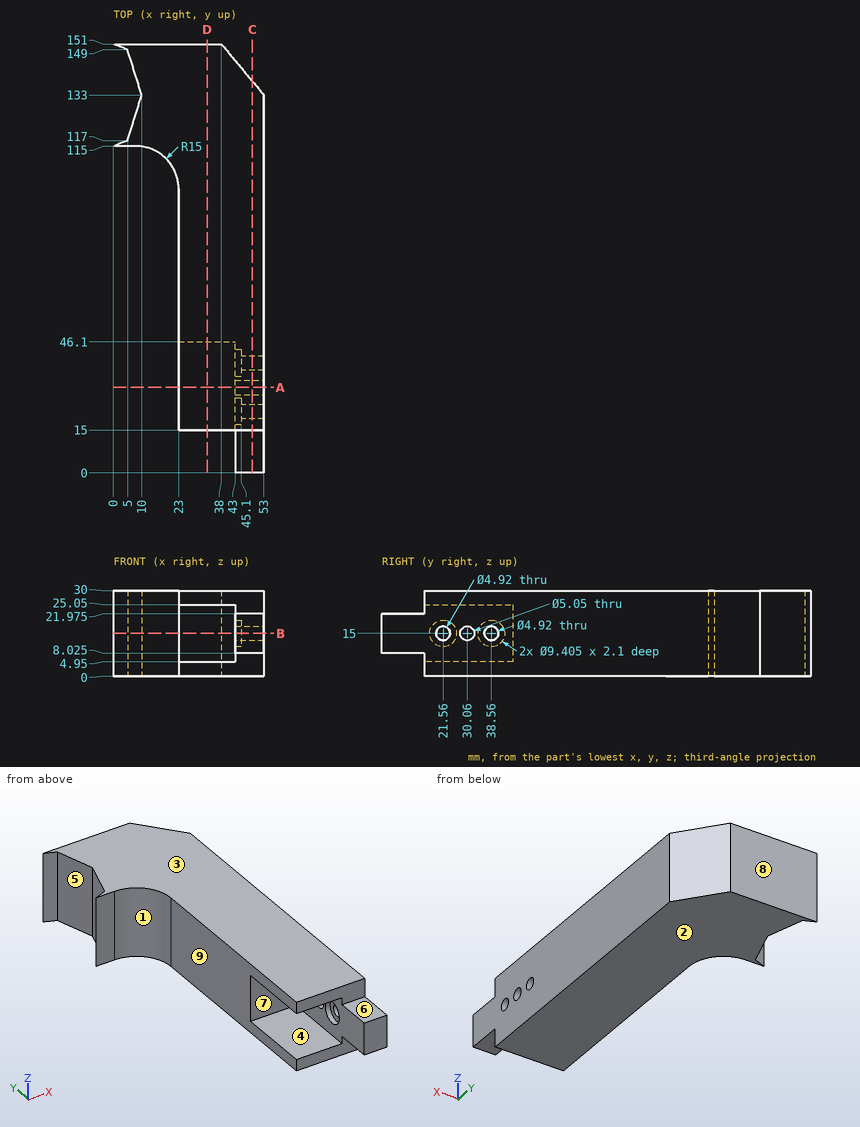
Answer from the drawing. Dimensions are ordinates in mm from the lowest x, y and z of the part. A direction names the side the tool comes from. Coordinates: 2 decimals unless noted, no trailing zeros. Order: outer loops, then holes, each group sorted by start corner. A loop starts at its lowest first (then second) coordinate and runs counter-clockwise, first axis right, second up. Notation, with made-up numbers: (79, 73) -> (92, 73) arc R15 cw to (92, 77) -> close; hole circle Ø11 at (16.25, 21.25). An arc over 180 degrees is marked (long way). Answer as a JSON object with one key per item and string values.
1) A cutting plane is placed at D-D, the plane x = 33. Determine the outline of the cut face in (y, z).
Model answer:
{"outline": "(15, 0) -> (151, 0) -> (151, 30) -> (15, 30) -> (15, 25.05) -> (46.1, 25.05) -> (46.1, 4.95) -> (15, 4.95) -> close"}
2) A tool of negligible diameter and unlimited length cuts with its end or side. For the marked faces 5, 6, 7, 8 and 9, from which of +Z, -Z, +X, -X, +Y, -Y can it reach the whole face along a straight path? Write none if from no direction.
Model answer:
{"face 5": "+Z, -Z, -X", "face 6": "+Z, +X, -X, -Y", "face 7": "-X, -Y", "face 8": "+Z, -Z, +X, -X, +Y", "face 9": "+Z, -Z, -X, -Y"}
3) Each of these flat-tipped pins is pushed along its axis until it touches: pin 1 (4.5 mm diameter, centred on y = 20.5, z = 16, fed in from -X); pin 2 (11 mm diameter, centred on y = 38.56, z = 15, fed in from -X); pin 3 (6 mm diameter, centred on x = 15, z = 5.5, fed in from -Y). Where does it stop, or does it pass through?
Model answer:
{"pin 1": "stops at x = 45.1", "pin 2": "stops at x = 43", "pin 3": "stops at y = 111.18"}
4) The mould has two halves that part along Z. Classify the marked faces 1, 2, 3 and 4: released by +Z, released by -Z, zero draft, split by the parting line, or undercut.
Model answer:
{"face 1": "zero draft", "face 2": "released by -Z", "face 3": "released by +Z", "face 4": "undercut"}
5) A cutting plane is placed at A-A, the plane y = 30.06. Determine the outline of the cut face in (x, z) (3 decimals), plus the area to 4 significant figures.
Model answer:
{"outline": "(23, 0) -> (53, 0) -> (53, 12.475) -> (43, 12.475) -> (43, 4.95) -> (23, 4.95) -> close; (23, 25.05) -> (43, 25.05) -> (43, 17.525) -> (53, 17.525) -> (53, 30) -> (23, 30) -> close", "area": "447.5 mm²"}
6) A cutting plane is placed at B-B, the plane z = 15. State how many separate pieces and enclosed holes the cut face has, plus the area to 3 significant figures.
Model answer:
{"separate pieces": "4", "enclosed holes": "0", "area": "3,930 mm²"}
7) Consider line 1 along Y through (x, z) = (47, 15) (3 decimals); line 2 along Z through (x, y) = (50, 30); line 3 along Y through (x, z) = (44.5, 15) (1 decimal). Determine where each line is inside the solid, lowest interval first. Write a range as from..to.
Model answer:
{"line 1": "y = 0..19.1, 24.02..27.535, 32.585..36.1, 41.02..140.2", "line 2": "z = 0..12.48, 17.52..30", "line 3": "y = 0..16.9, 26.3..27.5, 32.6..33.9, 43.3..143.2"}
8) A cutting plane is placed at C-C, the plane x = 49. Determine the outline of the cut face in (y, z) (3 decimals).
Model answer:
{"outline": "(0, 8.025) -> (15, 8.025) -> (15, 0) -> (137.8, 0) -> (137.8, 30) -> (15, 30) -> (15, 21.975) -> (0, 21.975) -> close; hole circle Ø4.92 at (21.56, 15); hole circle Ø5.05 at (30.06, 15); hole circle Ø4.92 at (38.56, 15)"}
